Check sheet for the modelled part. Datum: model origin and axes. Units: mm. A direction names the side the tool comes from. Coordinates: 2 decimals unless noted, no trailing zeros. Write each loop counter-clockwise with the first axis right and the second up, starting at its lowest first coordinate (ties: lowest second). Pieces come first, ordered by that corner, then holes. Notation, with made-up numbers: M -36,-38.5 L -2,-38.5 A28 cw -2,-17.5 Z; hole C -9.75,59.5 d4. An arc over 180 degrees is marked long. Answer as CSV lines item,"result". Start each with the question number.
Q1. Sectioned sample at C-C, the plane y = 16.25. Count the separate pieces of the cut face and the enclosed holes in it, then the cut area to 3 significant figures.
Q2. Access from +Z, -Z, +X, -X, +Y, -Y to the whole of each face (thin tool, end or side, straight path). Record for faces 1 (the cylindrical face through (20.947, 12.272, 1.524)), 2 (the cylindrical face through (-0.3, 9.4, 1.6)).
Q3. Sectioned sample at D-D, the plane x = 26.5. Record the cut outline in (y, z).
Q4. Mould release check, pull along X, two halves, no side actions. Record for faces 3 (the flat face through (21, 24.892, -3)), 4 (the cylindrical face through (-30.224, 12.272, 0.14)), 5 (the flat face through (0, 10, -3.048)): pulls with the +X half, pulls with the -X half, needs draft (parallel to the pull), parting line crosses it, or undercut.
Q5. Sectioned sample at B-B, the plane x = 0. Record the cut outline in (y, z).
Q6. Depth check by flat-ended pin: pin 1 Ø8 at (x, y) = (2.5, 16.5) entering from -Z. Enter the tip coordinate at first touch or a pass-through.
Q7. Sectioned sample at A-A, the plane z = 0. Record the cut outline in (x, y), then the cut area to 3 significant figures.
Q8. Thickness scan on line 1 along X through (y, z) = (15, 0); line 2 along X through (y, z) = (9, 0); line 3 along X through (y, z) = (11.5, 0). Record the ranges inside material, lowest first. Write a range as from..to.
from build123d import *

# Parameters (mm, degrees)
SKETCH1_R           = 3.302
BOSS_EXTRUDE1_DEPTH = 24.892
SKETCH2_R           = 16.002
CUT_EXTRUDE1_DEPTH  = 9.398
SKETCH3_R           = 14.986
CUT_EXTRUDE2_DEPTH  = 17.78
CHAMFER1_SIZE       = 0.254


with BuildPart() as part:
    # Sketch1 → Boss-Extrude1 (new body)
    with BuildSketch(Plane(origin=(0, 0, 0), x_dir=(1, 0, 0), z_dir=(0, 1, 0))):
        with BuildLine():
            Line((-23.876, 6.35), (23.876, 6.35))
            ThreePointArc((23.876, 6.35), (30.226, 0), (23.876, -6.35))
            Line((23.876, -6.35), (-23.876, -6.35))
            ThreePointArc((-23.876, -6.35), (-30.226, 0), (-23.876, 6.35))
        make_face()
        with Locations(Location((23.876, 0, 0), (0, 0, 270))):
            Circle(SKETCH1_R, mode=Mode.SUBTRACT)
        with Locations(Location((-23.876, 0, 0), (0, 0, 270))):
            Circle(SKETCH1_R, mode=Mode.SUBTRACT)
    extrude(amount=BOSS_EXTRUDE1_DEPTH)

    # Sketch2 → Cut-Extrude1 (cut)
    with BuildSketch(Plane.XY.offset(6.35)):
        with Locations((0, 25.4)):
            Circle(SKETCH2_R)
    extrude(amount=-CUT_EXTRUDE1_DEPTH, mode=Mode.SUBTRACT)

    # Sketch3 → Cut-Extrude2 (cut)
    with BuildSketch(Plane.XY.offset(-3.048)):
        with Locations((0, 25.4)):
            Circle(SKETCH3_R)
    extrude(amount=-CUT_EXTRUDE2_DEPTH, mode=Mode.SUBTRACT)

    # Chamfer1
    chamfer1_edges = [part.edges().sort_by_distance(p)[0] for p in [
        (0, 9.398, 6.35),
        (0, 10.414, -6.35),
    ]]
    chamfer(chamfer1_edges, length=CHAMFER1_SIZE)


solid = part.part
Output:
1,separate pieces,"2"
1,enclosed holes,"2"
1,area,"339 mm^2"
2,face 1,"+Y, -Y"
2,face 2,"+Z, +Y"
3,outline,"M 0,-5.78 L 24.89,-5.78 L 24.89,-2 L 0,-2 Z; M 0,2 L 24.89,2 L 24.89,5.78 L 0,5.78 Z"
4,face 3,"needs draft"
4,face 4,"pulls with the -X half"
4,face 5,"undercut"
5,outline,"M 0,-6.35 L 10.16,-6.35 L 10.41,-6.1 L 10.41,-3.05 L 9.4,-3.05 L 9.4,6.1 L 9.14,6.35 L 0,6.35 Z"
6,pin 1,"passes through"
7,outline,"M -30.23,0 L -27.18,0 L -27.18,24.89 L -30.23,24.89 Z; M -20.57,0 L 20.57,0 L 20.57,24.89 L 15.99,24.89 A16 cw -15.99,24.89 L -20.57,24.89 Z; M 27.18,0 L 30.23,0 L 30.23,24.89 L 27.18,24.89 Z"
7,area,"790 mm^2"
8,line 1,"x = -30.23..-27.18, -20.57..-12.16, 12.16..20.57, 27.18..30.23"
8,line 2,"x = -30.23..-27.18, -20.57..20.57, 27.18..30.23"
8,line 3,"x = -30.23..-27.18, -20.57..-7.93, 7.93..20.57, 27.18..30.23"
